For this review, take the finished solid that the model builds, in its own axes (mm). Face numbers are marked on the shaded views. A direction names the side the tool comes from. Give positions to 0.01 mm unless a question says otherwise; leave off trailing zeros. Loops run counter-clockwise (first coordinate to the right, second up) from the corner with the lowest first, then second, coordinate; pieces in that order, holes last. Notation, with made-up numbers: (76, 55) - (82, 55) arc R31 ccw to (82, 85) - close; hole circle Ø11 at (61.25, 65.25). An arc over 180 degrees is marked (long way). Answer in a Markdown table with one row per item.
```python
from build123d import *

# Parameters (mm, degrees)
ESBO_O1_R                = 21
RESSALTO_EXTRUS_O1_DEPTH = 46
FILETE1_R                = 10
ESBO_O2_R                = 3.079372868
RESSALTO_EXTRUS_O2_DEPTH = 16
ESBO_O3_R                = 2.5
RESSALTO_EXTRUS_O3_DEPTH = 29
RESSALTO_EXTRUS_O4_DEPTH = 10
ESBO_O5_R                = 21
CORTE_EXTRUS_O2_DEPTH    = 101.029128289
ESBO_O6_R                = 21
RESSALTO_EXTRUS_O5_DEPTH = 10
ESBO_O7_R                = 1.5
CORTE_EXTRUS_O3_DEPTH    = 101.029128289


with BuildPart() as part:
    # Esbo_o1 → Ressalto-extrus_o1 (new body)
    with BuildSketch(Plane.XY):
        with Locations((-33.295415682, 25.452495544)):
            Circle(ESBO_O1_R)
    extrude(amount=RESSALTO_EXTRUS_O1_DEPTH)

    # Filete1
    filete1_edges = [part.edges().sort_by_distance(p)[0] for p in [
        (-54.295415682, 25.452495544, 0),
        (-54.295415682, 25.452495544, 46),
    ]]
    fillet(filete1_edges, radius=FILETE1_R)

    # Esbo_o2 → Ressalto-extrus_o2 (add)
    with BuildSketch(Plane(origin=(0, 0, 0), x_dir=(-1, 0, 0), z_dir=(0, 0, -1))):
        with Locations(Location((33.295415682, 25.452495544, 0), (0, 0, 180))):
            Circle(ESBO_O2_R)
    extrude(amount=RESSALTO_EXTRUS_O2_DEPTH)

    # Esbo_o3 → Ressalto-extrus_o3 (add)
    with BuildSketch(Plane(origin=(0, 0, -16), x_dir=(-1, 0, 0), z_dir=(0, 0, -1))):
        with Locations((33.295415682, 25.452495544)):
            Circle(ESBO_O3_R)
    extrude(amount=RESSALTO_EXTRUS_O3_DEPTH)

    # Esbo_o4 → Ressalto-extrus_o4 (add)
    with BuildSketch(Plane.XY.offset(25)):
        Polygon((-33.295415682, 46.452495544), (-12.295415682, 46.452495544), (-12.295415682, 4.452495544), (-54.295415682, 4.452495544), (-54.295415682, 46.452495544), align=None)
    extrude(amount=RESSALTO_EXTRUS_O4_DEPTH)

    # Esbo_o5 → Corte-extrus_o2 (cut, through all)
    with BuildSketch(Plane.XY.offset(25)):
        with Locations(Location((-33.295415682, 25.452495544, 0), (0, 0, 180))):
            Circle(ESBO_O5_R)
    extrude(amount=CORTE_EXTRUS_O2_DEPTH, mode=Mode.SUBTRACT)


with BuildPart() as corte_extrus_o2_piece_1:
    # of the separate pieces the step leaves, piece 1, a body of its own (corte_extrus_o2_pieces)
    add(part.part.solids().sort_by_distance((-12.295415682, 25.452495544, 10))[0])



with BuildPart() as corte_extrus_o2_piece_2:
    # of the separate pieces the step leaves, piece 2, a body of its own (corte_extrus_o2_pieces)
    add(part.part.solids().sort_by_distance((-54.295415682, 46.452495544, 25))[0])


with BuildPart() as corte_extrus_o2_piece_3:
    # of the separate pieces the step leaves, piece 3, a body of its own (corte_extrus_o2_pieces)
    add(part.part.solids().sort_by_distance((-54.295415682, 4.452495544, 25))[0])


with BuildPart() as corte_extrus_o2_piece_4:
    # of the separate pieces the step leaves, piece 4, a body of its own (corte_extrus_o2_pieces)
    add(part.part.solids().sort_by_distance((-12.295415682, 46.452495544, 25))[0])


with BuildPart() as corte_extrus_o2_piece_5:
    # of the separate pieces the step leaves, piece 5, a body of its own (corte_extrus_o2_pieces)
    add(part.part.solids().sort_by_distance((-12.295415682, 4.452495544, 25))[0])


with BuildPart() as corte_extrus_o2_piece_1_1:
    add(corte_extrus_o2_piece_1.part)

    add(corte_extrus_o2_piece_2.part)  # Ressalto-extrus_o5 merges Corte-extrus_o2 piece 2

    add(corte_extrus_o2_piece_3.part)  # Ressalto-extrus_o5 merges Corte-extrus_o2 piece 3

    add(corte_extrus_o2_piece_4.part)  # Ressalto-extrus_o5 merges Corte-extrus_o2 piece 4

    add(corte_extrus_o2_piece_5.part)  # Ressalto-extrus_o5 merges Corte-extrus_o2 piece 5
    # Esbo_o6 → Ressalto-extrus_o5 (add)
    with BuildSketch(Plane.XY.offset(25)):
        with Locations((-33.295415682, 25.452495544)):
            Circle(ESBO_O6_R)
    extrude(amount=RESSALTO_EXTRUS_O5_DEPTH)

    # Esbo_o7 → Corte-extrus_o3 (cut, through all)
    with BuildSketch(Plane(origin=(0, 0, 25), x_dir=(-1, 0, 0), z_dir=(0, 0, -1))):
        with Locations((15.295415682, 43.452495544)):
            Circle(ESBO_O7_R)
        with Locations((51.295415682, 43.452495544)):
            Circle(ESBO_O7_R)
        with Locations((51.295415682, 7.452495544)):
            Circle(ESBO_O7_R)
        with Locations((15.295415682, 7.452495544)):
            Circle(ESBO_O7_R)
    extrude(amount=-CORTE_EXTRUS_O3_DEPTH, mode=Mode.SUBTRACT)


solid = corte_extrus_o2_piece_1_1.part
```
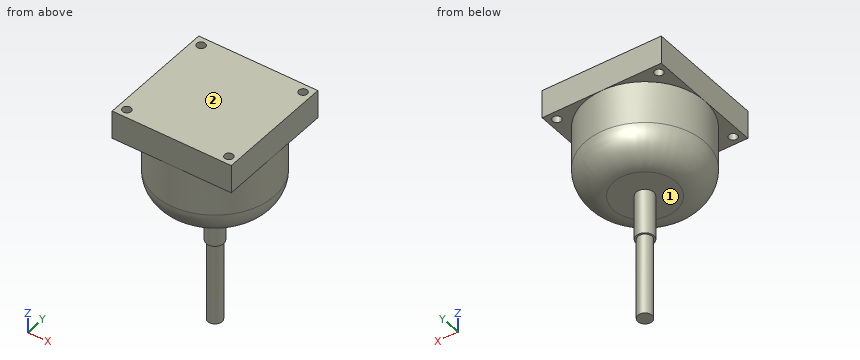
1. Wall thickness on line 1 (Y direction, x = -16.5, z = 30.5); line 2 (Z direction, x = -32.5, y = 22); line 3 (Z direction, x = -15, y = 41): over which ranges is each line inside the solid? List them lowest first. Write a range as [from, to].
Values:
| item | result |
|---|---|
| line 1 | y = [4.45, 6.56], [8.35, 42.56], [44.35, 46.45] |
| line 2 | z = [0, 35] |
| line 3 | z = [25, 35] |
2. Clearance check with flat-ended pins moving along their axes: pin 1 (3.5 mm diameter, centred on x = -15.3, y = 43.45, fed in from -Z); pin 2 (23 mm diameter, centred on x = -41.5, y = 41, fed in from -Z); pin 3 (4 mm diameter, centred on x = -29, z = 13.5, fed in from -Y). State where each tip first meets the part, or that it passes through.
Values:
| item | result |
|---|---|
| pin 1 | stops at z = 25 |
| pin 2 | stops at z = 0 |
| pin 3 | stops at y = 4.58 |
3. We need section C-C, the plane z = -23.5. Give the boundary of the cut face in (x, y).
Values:
| item | result |
|---|---|
| outline | circle Ø5 at (-33.3, 25.45) |
4. We need section B-B, the plane x = -15. Count the separate pieces of the cut face and the enclosed holes in it, and give its area (3 significant figures).
Values:
| item | result |
|---|---|
| separate pieces | 3 |
| enclosed holes | 0 |
| area | 782 mm^2 |
5. We need section D-D, the plane z = 4.5. Give the boundary of the cut face in (x, y), and give its area (3 significant figures).
Values:
| item | result |
|---|---|
| outline | circle Ø38.7 at (-33.3, 25.45) |
| area | 1,180 mm^2 |
6. For the marked faces 1 and 2, list the 3-axis set-ups (+Z, -Z, +X, -X, +Y, -Y) from which the entire face can be reached by the end or side of a thin tool; tool diameter is ignored.
Values:
| item | result |
|---|---|
| face 1 | -Z |
| face 2 | +Z, +X, -X, +Y, -Y |
7. We need section A-A, the plane z = 27. Give the boundary of the cut face in (x, y).
Values:
| item | result |
|---|---|
| outline | (-54.3, 4.45) - (-12.3, 4.45) - (-12.3, 46.45) - (-54.3, 46.45) - close; hole circle Ø3 at (-51.3, 7.45); hole circle Ø3 at (-51.3, 43.45); hole circle Ø3 at (-15.3, 7.45); hole circle Ø3 at (-15.3, 43.45) |
